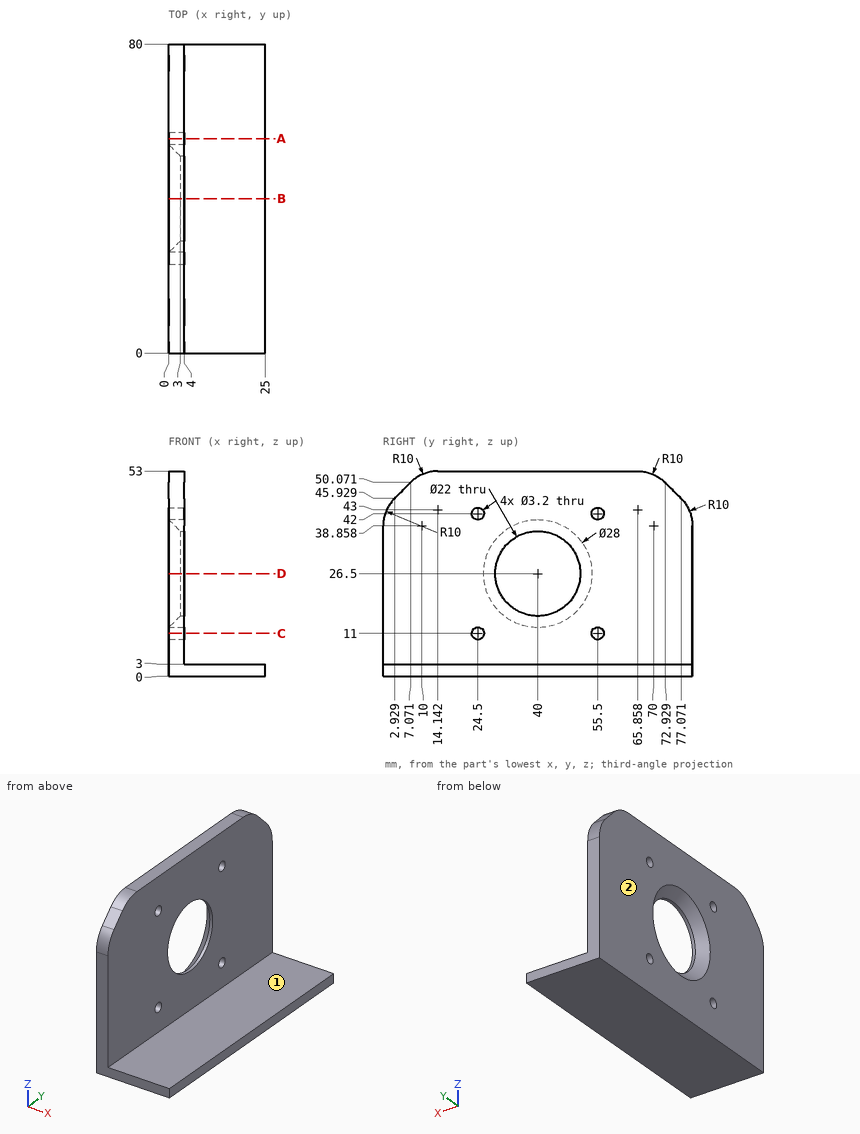
Part print with two shaded views. Sizes in mm from the minimum x, y, z corner. A direction names the side the tool comes from. Coordinates: 2 decimals unless noted, no trailing zeros. Loops run counter-clockwise (first coordinate to the right, second up) from the corner with the lowest first, then second, coordinate; pieces in that order, holes last. Notation, with made-up numbers: (40.5, -22.75) - (98.5, -22.75) arc R9 cw to (98.5, -10.75) - close; hole circle Ø11 at (86, -13). An arc over 180 degrees is marked (long way). Write each question's results on one line, items separated by ' | '. Start each with the question number.
Q1. Which spindle directions (+Z, -Z, +X, -X, +Y, -Y) get a long thin tool onto all of the face, cutting with end or side? Do the marked faces 1 and 2. Say none if no direction does.
Q2. Slice it at A-A on y = 55.5. Give the cut face in (x, z), and give its area (3 significant figures).
Q3. Slice it at D-D on z = 26.5. Give the cut face in (x, y), and give its area (3 significant figures).
Q4. Slice it at C-C on z = 11. Give the cut face in (x, y).
Q5. Drop flat-ended pins along their axis: pin 1 Ø4 at (y, z) = (30.5, 32) entering from -X; pin 2 Ø10.5 at (x, y) = (12, 22.5) entering from +Z; pin 3 Ø6 at (y, z) = (29, 17) entering from +X. Give the stop position or say it passes through.
Q6. Slice it at B-B on y = 40. Give the cut face in (x, z), and give its area (3 significant figures).
Q7. Probe line 1 along Y through (x, z) = (3.5, 26.5); line 2 along Y through (x, z) = (2.8, 42); line 3 along X through (y, z) = (9, 26). List the from-to ranges inside material, lowest first.
Answer:
1) face 1: +Z, +X, +Y, -Y | face 2: +Z, -Z, -X, +Y, -Y
2) outline: (0, 0) - (25, 0) - (25, 3) - (4, 3) - (4, 9.4) - (0, 9.4) - close; (0, 12.6) - (4, 12.6) - (4, 40.4) - (0, 40.4) - close; (0, 43.6) - (4, 43.6) - (4, 53) - (0, 53) - close | area: 249 mm2
3) outline: (0, 0) - (4, 0) - (4, 29) - (3, 29) - (0, 26) - close; (0, 54) - (3, 51) - (4, 51) - (4, 80) - (0, 80) - close | area: 223 mm2
4) outline: (0, 0) - (4, 0) - (4, 22.9) - (0, 22.9) - close; (0, 26.1) - (4, 26.1) - (4, 53.9) - (0, 53.9) - close; (0, 57.1) - (4, 57.1) - (4, 80) - (0, 80) - close
5) pin 1: stops at x = 1.02 | pin 2: stops at z = 3 | pin 3: stops at x = 4
6) outline: (0, 0) - (25, 0) - (25, 3) - (4, 3) - (4, 15.5) - (3, 15.5) - (0, 12.5) - close; (0, 40.5) - (3, 37.5) - (4, 37.5) - (4, 53) - (0, 53) - close | area: 178 mm2
7) line 1: y = 0 to 29, 51 to 80 | line 2: y = 0.51 to 22.9, 26.1 to 53.9, 57.1 to 79.49 | line 3: x = 0 to 4
